Work out the finished part from the listing and answer in its coordinate system (mm). A direction names the side the tool comes from. Coordinates: 2 decimals unless noted, no trailing zeros. Order: outer loops, then holes, each group sorted by start corner. A loop starts at its lowest first (then second) coordinate and runs counter-clockwise, first axis right, second up. Notation, with made-up numbers: M -38,78.5 L -26,78.5 A28 ccw -26,100.5 Z; hole C 47.25,74 d10. An arc over 180 degrees is marked long. Write item = value, one per line. Start each with the question number.
Q1. A tool of negligible diameter and unlimited length cuts with its end or side. For faces 1 (the cylindrical face through (1.565, 12.588, 142.238)), 2 (the flat face through (22.225, 13, 88)), from which of +Z, -Z, +X, -X, +Y, -Y can it reach the whole face along a straight path? Write none if from no direction.
Q2. Find section B-B on y = 23.75. Give the vertices of the cut face in (x, z) (3 decimals).
Q3. Find section A-A on z = 139.7. Give the vertices of the cut face in (x, y) (3 decimals), and give its area (3 significant figures).
Q4. This flat-tipped pin is pushed along its axis until it touches: P1, Ø4, axis at y = 12.7, z = 12.7, coming from the +X side (1 decimal). Where does it stop, or does it pass through?
Q5. Find section D-D on z = 118. Give the vertices of the cut face in (x, y) (3 decimals), and give its area (3 significant figures).
Q6. Straight lines are drawn through the part: line 1 along Z through (x, y) = (12.7, 0.75) (3 decimals); line 2 along Y through (x, z) = (9.25, 100) (3 decimals); line 3 along X through (y, z) = (1, 38.1) (3 decimals). For each, find the intervals that lie inside material, in ascending order.
Q7. Find section C-C on x = 18.25. Give the vertices of the cut face in (y, z) (3 decimals), and give its area (3 significant figures).
Q8. Determine the mould class of faces 3 (the cylindrical face through (23.79, 12.588, 142.238)), 4 (the flat face through (13, 0, 88)), 5 (the flat face through (13, 25.4, 88)), 6 (the cylindrical face through (12.56, 23.79, 34.93)) for opening direction Y: released by +Y, released by -Y, zero draft, split by the parting line, or undercut.
Autodesk Inventor part; units mm, degrees
ref_plane "YZ Plane" through (0, 0, 0) normal (1, 0, 0) x (0, 1, 0)
ref_plane "XZ Plane" through (0, 0, 0) normal (0, 1, 0) x (-1, 0, 0)
ref_plane "XY Plane" through (0, 0, 0) normal (0, 0, 1) x (1, 0, 0)
sketch "Sketch1" plane through (0, 0, 0) normal (0, 0, 1) x (1, 0, 0)
  line L0 (0, 0) -> (25.4, 0)
  line L1 (25.4, 0) -> (25.4, 25.4)
  line L2 (25.4, 25.4) -> (0, 25.4)
  line L3 (0, 25.4) -> (0, 0)
  line L4 (22.225, 22.225) -> (22.225, 3.175)
  line L5 (22.225, 3.175) -> (3.175, 3.175)
  line L6 (3.175, 3.175) -> (3.175, 22.225)
  line L7 (3.175, 22.225) -> (22.225, 22.225)
  dimension "d0" = 25.4
  dimension "d1" = 25.4
  dimension "d2" = 3.175
extrude "Extrusion1" add sketch "Sketch1" along normal blind 177.8
sketch "Sketch2" plane through (0, 25.4, 0) normal (0, 1, 0) x (1, 0, 0)
  line L0 (25.4, 0) -> (25.4, -177.8)
  line L1 (25.4, -177.8) -> (0, -177.8)
  line L2 (25.4, 0) -> (0, 0)
  line L3 (0, 0) -> (0, -177.8)
  point P0 (12.7, -165.1)
  point P1 (12.7, -12.7)
  dimension "d5" = 12.7
  dimension "d6" = 12.7
  dimension "d7" = 12.7
  dimension "d8" = 12.7
hole "Hole1" at (12.7, 25.4, 165.1) at (12.7, 25.4, 12.7) direction (0, -1, 0) diameter 6.35 end through all
pattern_linear "Rectangular Pattern1" count 2 spacing 25.4 along (0, 0, 1) count 2 spacing 25.4 along (0, 0, -1) of "Hole1"
sketch "Sketch4" plane through (25.4, 0, 0) normal (1, 0, 0) x (0, 0, -1)
  line L0 (0, 25.4) -> (-177.8, 25.4)
  line L1 (-177.8, 0) -> (-177.8, 25.4)
  line L2 (0, 0) -> (0, 25.4)
  point P0 (-165.1, 12.7)
  point P1 (-12.7, 12.7)
  dimension "d31" = 12.7
  dimension "d32" = 12.7
  dimension "d33" = 12.7
  dimension "d34" = 12.7
hole "Hole3" at (25.4, 12.7, 165.1) at (25.4, 12.7, 12.7) direction (-1, 0, 0) diameter 5.08 end through all
pattern_linear "Rectangular Pattern2" count 2 spacing 25.4 along (0, 0, -1) count 2 spacing 25.4 along (0, 0, 1) of "Hole3"
equation "\"d0\" = d1"
properties part number "testRoboRescue_Chassis_Frame_lengthBar" material "Aluminum 6061"
Findings below:
q1.face_1 = +X, -X
q1.face_2 = +Z, -Z
q2.outline = M 0,0 L 25.4,0 L 25.4,177.8 L 0,177.8 Z; hole C 12.7,12.7 d6.35; hole C 12.7,38.1 d6.35; hole C 12.7,139.7 d6.35; hole C 12.7,165.1 d6.35
q3.outline = M 0,0 L 9.525,0 L 9.525,3.175 L 3.175,3.175 L 3.175,10.16 L 0,10.16 Z; M 0,15.24 L 3.175,15.24 L 3.175,22.225 L 9.525,22.225 L 9.525,25.4 L 0,25.4 Z; M 15.875,0 L 25.4,0 L 25.4,10.16 L 22.225,10.16 L 22.225,3.175 L 15.875,3.175 Z; M 15.875,22.225 L 22.225,22.225 L 22.225,15.24 L 25.4,15.24 L 25.4,25.4 L 15.875,25.4 Z
q3.area = 210 mm^2
q4.P1 = through
q5.outline = M 0,0 L 25.4,0 L 25.4,25.4 L 0,25.4 Z; hole M 3.175,3.175 L 22.225,3.175 L 22.225,22.225 L 3.175,22.225 Z
q5.area = 282 mm^2
q6.line_1 = 0 to 9.525, 15.875 to 34.925, 41.275 to 136.525, 142.875 to 161.925, 168.275 to 177.8
q6.line_2 = 0 to 3.175, 22.225 to 25.4
q6.line_3 = 0 to 9.525, 15.875 to 25.4
q7.outline = M 0,0 L 3.175,0 L 3.175,177.8 L 0,177.8 Z; M 22.225,0 L 25.4,0 L 25.4,177.8 L 22.225,177.8 Z
q7.area = 1,130 mm^2
q8.face_3 = undercut
q8.face_4 = released by -Y
q8.face_5 = released by +Y
q8.face_6 = zero draft
